Part model, mm, in its own coordinate system. A direction names the side the tool comes from. Coordinates: 2 decimals unless noted, no trailing zeros. Write each loop counter-clockwise with the first axis right and the second up, starting at its lowest first coordinate (ties: lowest second). Pieces come first, ordered by that corner, then holes. Notation, with made-up numbers: (47.25, 18.25) - (96.25, 18.25) arc R21 cw to (96.25, 30.25) - close; hole circle Ø4 at (23, -25). An arc over 180 degrees is marked (long way). Use a Markdown table: item, result.
```python
from build123d import *

# Parameters (mm, degrees)
F3_R = 3.175


with BuildPart() as f2:
    # F2: sweep along a path in F1
    with BuildLine(Plane.XZ) as f2_path:
        Line((25.4, 0), (25.4, 38.1))
        Line((25.4, 38.1), (43.3605122421, 56.0605122421))
        Line((43.3605122421, 56.0605122421), (43.3605122421, 68.7605122421))
    # F0 (on Top) → F2 (sweep)
    with BuildSketch(Plane.XY):
        with BuildLine():
            Line((50.8, 0), (0, 0))
            Line((0, 0), (0, -25.4))
            Line((0, -25.4), (25.4, -25.4))
            ThreePointArc((25.4, -25.4), (68.7605122421, -43.3605122421), (50.8, 0))
        make_face()
    sweep(path=f2_path.line, transition=Transition.RIGHT)

    # F3
    f3_edges = [f2.edges().sort_by_distance(p)[0] for p in [
        (8.980256, -25.4, 57.601281),
        (0, -25.4, 24.310512),
        (0, -12.7, 48.621024),
        (0, 0, 24.310512),
        (8.980256, 0, 57.601281),
        (17.960512, -25.4, 67.671024),
        (30.660512, -25.4, 68.760512),
        (17.960512, 0, 67.671024),
        (43.360512, 0, 68.760512),
    ]]
    fillet(f3_edges, radius=F3_R)


solid = f2.part
```
Item 1: Drop flat-ended pins along their axis: P1, Ø5, axis at y = -16.5, z = 11.5, coming from the +X side; P2, Ø6, axis at y = -24.5, z = 49.5, coming from the -X side; P3, Ø12, axis at y = -24, z = 7.5, coming from the +X side; P4, Ø2, axis at x = 31, y = -44.5, coming from the +Z side. Give the stop position or say it passes through.
From the geometry:
| item | result |
|---|---|
| P1 | x = 75.38 |
| P2 | x = 0 |
| P3 | x = 76.2 |
| P4 | through |
Item 2: Which spindle directions (+Z, -Z, +X, -X, +Y, -Y) get a long thin tool onto all of the face, cutting with end or side? Do faces 1 (the face through (17.961, -13, 68)), 2 (the face through (56.56, -50.14, 15.08)), 3 (the face through (18.55, -1.33, 67.04)). Say none if no direction does.
From the geometry:
| item | result |
|---|---|
| face 1 | +Z, -X, +Y, -Y |
| face 2 | -Z |
| face 3 | +Z, -X, +Y |
Item 3: Band-saw the part on A-A, the plane z = 6. Give the cut face in (x, y) (3 decimals).
From the geometry:
| item | result |
|---|---|
| outline | (0, -22.225) arc R3.175 ccw to (3.175, -25.4) - (25.4, -25.4) arc R25.4 ccw (long way) to (50.8, 0) - (3.175, 0) arc R3.175 ccw to (0, -3.175) - close |
Item 4: Drill centre lines: probe 1 along Y at (x, z) = (15, 36); probe 2 along X at (y, z) = (-47, 33); probe 3 along Z at (x, y) = (43, -30.5). Where is each one in solid material? Low to high.
From the geometry:
| item | result |
|---|---|
| probe 1 | -25.4 to 0 |
| probe 2 | 37.44 to 75.12 |
| probe 3 | 0 to 54.97 |
